Geometry check sheet. Reference: the model listing, model coordinates, mm. Give positions to 0.01 mm unless a question says otherwise; leave off trailing zeros. Order: outer loops, then holes, each group sorted by start corner. A loop starts at its lowest first (then second) coordinate and runs counter-clockwise, first axis right, second up.
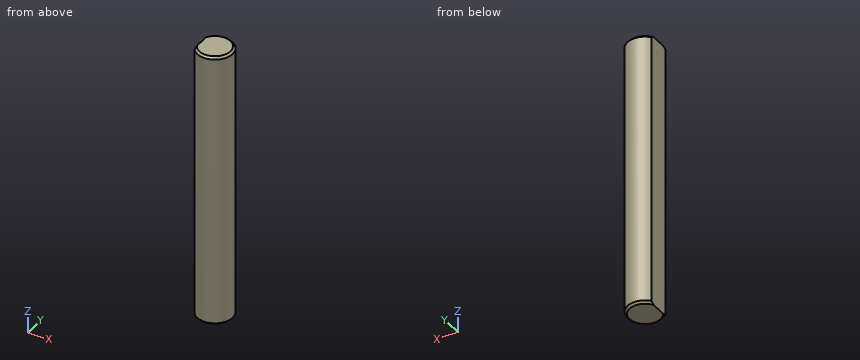
from build123d import *

# Parameters (mm, degrees)
SKETCH1_R           = 4.15
BOSS_EXTRUDE1_DEPTH = 65
CHAMFER1_SIZE       = 0.5
SKETCH2_W           = 1.287128146
SKETCH2_H           = 7.63924008
CUT_EXTRUDE1_DEPTH  = 33


with BuildPart() as part:
    # Sketch1 → Boss-Extrude1 (new body)
    with BuildSketch(Plane.XY):
        Circle(SKETCH1_R)
    extrude(amount=BOSS_EXTRUDE1_DEPTH)

    # Chamfer1
    chamfer1_edges = [part.edges().sort_by_distance(p)[0] for p in [
        (-4.15, 0, 0),
        (-4.15, 0, 65),
    ]]
    chamfer(chamfer1_edges, length=CHAMFER1_SIZE)

    # Sketch2 → Cut-Extrude1 (cut, symmetric)
    with BuildSketch(Plane.XY.offset(32.5)):
        with Locations((-3.793564073, 0)):
            Rectangle(SKETCH2_W, SKETCH2_H)
    extrude(amount=CUT_EXTRUDE1_DEPTH, both=True, mode=Mode.SUBTRACT)


solid = part.part
Item 1: Sectioned sample at A-A (z = 29.5). Enter the section's corners in (x, y).
Reported:
outline: (-3.15, -2.7) arc R4.15 ccw (long way) to (-3.15, 2.7) - close
Item 2: Scan lines: L1, parallel to X at y = 0.25, z = 61.5; L2, parallel to Y at x = -2, z = 14.5; L3, parallel to Y at x = -1.75, z = 43.5. Record each from-to range of solid material in increasing order.
Reported:
L1: x = -3.15 to 4.14
L2: y = -3.64 to 3.64
L3: y = -3.76 to 3.76
Item 3: Gauge pin test, flat end, axial feed: pin 1 (1 mm diameter, centred on y = 1, z = 23, fed in from +X). Record the tip position at first contact, or that the pin passes through.
Reported:
pin 1: stops at x = 4.12
